Part model, mm, in its own coordinate system. Face numbers are marked on the shaded views. Coordinates: 2 decimals unless noted, no trailing zeros. Loops run counter-clockwise (first coordinate to the right, second up) from the corner with the lowest first, then second, coordinate; pieces in that order, holes last. Notation, with made-up numbers: M 41.25,79 L 95.25,79 A18 ccw 95.25,88 Z; hole C 30,17.5 d1. An arc over 180 degrees is marked long. Answer as a JSON object with one key per item and string values. Group by question number.
1. Saw through at B-B on z = 124.5. Write the cut outline in (x, y), then the cut area to 3 significant figures.
2. Saw through at A-A on y = 0. Write the cut outline in (x, z).
3. Drill centre lines: L1, parallel to Y at x = 0, z = 50; L2, parallel to X at y = -6.5, z = 14.5; L3, parallel to X at y = 5, z = 92. Where is each one in solid material? Low to high.
4. Saw through at C-C on x = 0. Write the cut outline in (y, z), then the cut area to 3 significant figures.
5. Drop flat-ended pins along their axis: pin 1 Ø5 at (y, z) = (-4.5, 51) entering from +X; pin 2 Ø3 at (y, z) = (-8.5, 123) entering from -X; pin 3 Ø1.5 at (x, z) = (-9, 111) entering from +Y. Give the stop position or say it passes through.
6. Mould opens along Y. For the marked faces 1 and 2 say: released by +Y, released by -Y, zero draft, split by the parting line, or undercut.
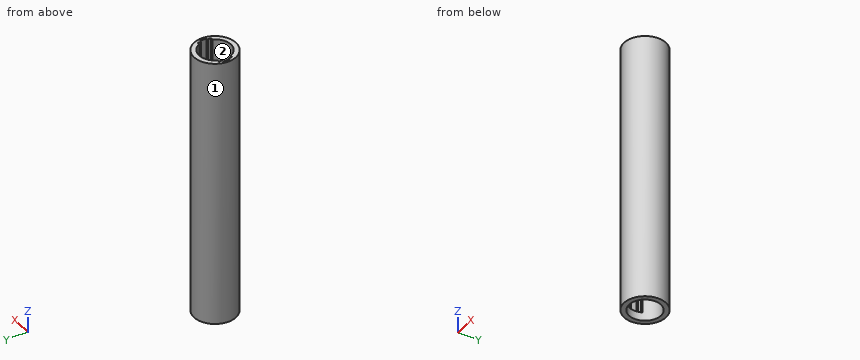
Autodesk Fusion 360 part; units mm, degrees
sketch "Sketch1" plane through (0, 0, 0) normal (0, 0, 1) x (1, 0, 0)
  circle A0 centre (0, 0) radius 12.5
  dimension "d1" = 25
extrude "Extrude1" add sketch "Sketch1" along normal blind 160
sketch "Sketch3" plane through (0, 0, 160) normal (0, 0, 1) x (-1, 0, 0)
  circle A0 centre (0, 0) radius 12.5
  circle A1 centre (0, 0) radius 9.5
  dimension "d4" = 19
extrude "Extrude2" cut sketch "Sketch3" against normal blind 1000 contours A1
sketch "Sketch4" plane through (0, 0, 160) normal (0, 0, -1) x (1, 0, 0)
  circle A0 centre (0, -30) radius 12.5
  circle A1 centre (0, -30) radius 9.25
  dimension "d12" = 18.5
sketch "Sketch7" plane through (0, 0, 171) normal (0, 0, 1) x (-1, 0, 0)
  circle A0 centre (30, 0) radius 6.2204
  circle A1 centre (30, 0) radius 5
sketch "Sketch8" plane through (0, 0, 171) normal (0, 0, 1) x (-1, 0, 0)
  circle A0 centre (30, 0) radius 5
  circle A1 centre (30, 0) radius 6.2204
  line L0 (26, -15) -> (14, -15)
  circle A2 centre (20, -15) radius 6
  line L1 (26, -20) -> (21, -20)
  line L2 (21, -10) -> (26, -10)
  line L3 (26, -10) -> (26, -20)
sketch "Sketch9" plane through (-26, 0, 0) normal (-1, 0, 0) x (0, -1, 0)
  circle A0 centre (-15, 171) radius 5
sketch "Sketch10" plane through (-26, 0, 0) normal (-1, 0, 0) x (0, -1, 0)
  circle A0 centre (-15, 171) radius 4
sketch "Sketch11" plane through (0, 0, 160) normal (0, 0, 1) x (-1, 0, 0)
  circle A0 centre (0, 0) radius 9.5
  circle A1 centre (0, 0) radius 12.5
  line L0 (11, 2) -> (-11, 2)
  line L1 (-11, 2) -> (-11, -2)
  line L2 (-11, -2) -> (11, -2)
  line L3 (11, -2) -> (11, 2)
  line L4 (10, -4) -> (-10, -4)
  line L5 (-10, -4) -> (-10, 4)
  line L6 (-10, 4) -> (10, 4)
  line L7 (10, 4) -> (10, -4)
extrude "Extrude7" cut sketch "Sketch11" against normal blind 155 contours A0 L0 L2 L7 | A0 L0 L6 L7 | A0 L2 L4 L7 | L0 L2 L3 L7 | A0 L0 L5 L6 | A0 L0 L2 L5 | A0 L2 L4 L5 | L0 L1 L2 L5
sketch "Sketch12" plane through (0, 0, 160) normal (0, 0, 1) x (-1, 0, 0)
  line L0 (11, -2) -> (10, -2)
  arc A0 (8.6168, 4) -> (-8.6168, 4) centre (0, 0) ccw
  line L1 (-10, -2) -> (-11, -2)
  line L2 (-11, -2) -> (-11, 2)
  line L3 (-11, 2) -> (-10, 2)
  line L4 (10, 2) -> (11, 2)
  line L5 (11, 2) -> (11, -2)
  circle A1 centre (0, 0) radius 12.5
  line L6 (10.9, -1.9) -> (-10.9, -1.9)
  line L7 (-10.9, -1.9) -> (-10.9, 1.9)
  line L8 (-10.9, 1.9) -> (10.9, 1.9)
  line L9 (10.9, 1.9) -> (10.9, -1.9)
  line L10 (10, -3) -> (-10, -3)
  line L11 (-10, -3) -> (-10, 3)
  line L12 (-10, 3) -> (10, 3)
  line L13 (10, 3) -> (10, -3)
  line L14 (-8.6168, -4) -> (-10, -4)
  line L15 (-10, -4) -> (-10, -2)
  line L16 (-10, 2) -> (-10, 4)
  line L17 (-10, 4) -> (-8.6168, 4)
  line L18 (8.6168, 4) -> (10, 4)
  line L19 (10, 4) -> (10, 2)
  line L20 (10, -2) -> (10, -4)
  line L21 (10, -4) -> (8.6168, -4)
  arc A2 (-8.6168, -4) -> (8.6168, -4) centre (0, 0) ccw
sketch "Sketch13" plane through (0, -1.9, 0) normal (0, -1, 0) x (1, 0, 0)
  line L0 (37.9, 160) -> (16.1, 160)
  line L1 (16.1, 160) -> (16.1, 0)
  line L2 (16.1, 0) -> (37.9, 0)
  line L3 (37.9, 0) -> (37.9, 160)
  line L4 (18, 158) -> (36, 158)
  line L5 (36, 158) -> (36, 16)
  line L6 (36, 16) -> (18, 16)
  line L7 (18, 16) -> (18, 158)
sketch "Sketch14" plane through (0, -1.9, 0) normal (0, -1, 0) x (1, 0, 0)
  line L0 (16, 0) -> (19.1, 0)
  line L1 (19.1, 0) -> (19.1, 5.1)
  line L2 (19.1, 5.1) -> (16, 5.1)
  line L3 (16, 5.1) -> (16, 0)
  line L4 (38, 0) -> (34.9, 0)
  line L5 (34.9, 0) -> (34.9, 5.1)
  line L6 (34.9, 5.1) -> (38, 5.1)
  line L7 (38, 5.1) -> (38, 0)
sketch "Sketch15" plane through (0, 0, 0) normal (0, 0, -1) x (1, 0, 0)
  line L0 (19.1, 1.9) -> (19.1, -1.9)
  line L1 (19.1, -1.9) -> (34.9, -1.9)
  line L2 (34.9, -1.9) -> (34.9, 1.9)
  line L3 (34.9, 1.9) -> (19.1, 1.9)
  circle A0 centre (27, 0) radius 7.9
  circle A1 centre (27, 0) radius 7.6941
Outcome:
{
 "1": {"outline": "C 0,0 d25; hole M -11,-2 L -10,-2 L -10,-4 L -8.62,-4 A9.5 ccw 8.62,-4 L 10,-4 L 10,-2 L 11,-2 L 11,2 L 10,2 L 10,4 L 8.62,4 A9.5 ccw -8.62,4 L -10,4 L -10,2 L -11,2 Z", "area": "187 mm²"},
 "2": {"outline": "M -12.5,0 L -9.5,0 L -9.5,5 L -11,5 L -11,160 L -12.5,160 Z; M 9.5,0 L 12.5,0 L 12.5,160 L 11,160 L 11,5 L 9.5,5 Z"},
 "3": {"L1": "y = -12.5 to -9.5, 9.5 to 12.5", "L2": "x = -10.68 to -6.93, 6.93 to 10.68", "L3": "x = -11.46 to -8.08, 8.08 to 11.46"},
 "4": {"outline": "M -12.5,0 L -9.5,0 L -9.5,160 L -12.5,160 Z; M 9.5,0 L 12.5,0 L 12.5,160 L 9.5,160 Z", "area": "960 mm²"},
 "5": {"pin 1": "stops at x = 12.34", "pin 2": "stops at x = -10.36", "pin 3": "stops at y = 9.39"},
 "6": {"face 1": "split by the parting line", "face 2": "undercut"}
}
